Design review of the part built by this model. Coordinates are the model's own, in mm. A direction names the side the tool comes from. Give positions to 0.01 mm unless a question says otherwise; leave off trailing zeros. Write each loop counter-clockwise with the first axis right and the second up, starting at its lowest first coordinate (ties: lowest second). Pieces come first, ordered by that corner, then holes. Notation, with made-up numbers: M 83,-17 L 96,-17 A31 cw 96,20 Z; hole C 84,73 d4. An arc over 180 degrees is marked long. Answer in a Markdown table with one row per item.
```python
from build123d import *

# Parameters (mm, degrees)
EXTRUDE_1_DEPTH     = 10
FILLET_1_R          = 10
CUT_EXTRUDE_1_DEPTH = 211.475651798
CUT_EXTRUDE_2_DEPTH = 7
SKETCH_4_W          = 20.2
SKETCH_4_H          = 40
CUT_EXTRUDE_3_DEPTH = 7
CUT_EXTRUDE_4_DEPTH = 7


with BuildPart() as part:
    # Эскиз1 → Бобышка-Вытянуть1 (new body)
    with BuildSketch(Plane.XY):
        Polygon((0, 0), (60, 0), (60, -60), (90, -70.919107028), (90, -129.080892972), (60, -140), (60, -180), (0, -180), (0, -140), (-30, -129.080892972), (-30, -70.919107028), (0, -60), align=None)
    extrude(amount=EXTRUDE_1_DEPTH)

    # Скругление1
    fillet_1_edges = [part.edges().sort_by_distance(p)[0] for p in [
        (60, -60, 5),
        (90, -70.919107028, 5),
        (90, -129.080892972, 5),
        (60, -140, 5),
        (60, -180, 5),
        (0, -180, 5),
        (0, -140, 5),
        (-30, -129.080892972, 5),
        (-30, -70.919107028, 5),
        (0, -60, 5),
    ]]
    fillet(fillet_1_edges, radius=FILLET_1_R)

    # Эскиз2 → Вырез-Вытянуть1 (cut, through all)
    with BuildSketch(Plane(origin=(0, 10, 10), x_dir=(-1, 0, 0), z_dir=(0, 0, 1))):
        with BuildLine():
            Line((20, 102.25), (-80, 102.25))
            ThreePointArc((-80, 102.25), (-83.25, 99), (-80, 95.75))
            Line((-80, 95.75), (20, 95.75))
            ThreePointArc((20, 95.75), (23.25, 99), (20, 102.25))
        make_face()
        with BuildLine():
            Line((20, 91.25), (-80, 91.25))
            ThreePointArc((-80, 91.25), (-83.25, 88), (-80, 84.75))
            Line((-80, 84.75), (20, 84.75))
            ThreePointArc((20, 84.75), (23.25, 88), (20, 91.25))
        make_face()
        with BuildLine():
            Line((20, 113.25), (-80, 113.25))
            ThreePointArc((-80, 113.25), (-83.25, 110), (-80, 106.75))
            Line((-80, 106.75), (20, 106.75))
            ThreePointArc((20, 106.75), (23.25, 110), (20, 113.25))
        make_face()
        with BuildLine():
            Line((20, 124.25), (-80, 124.25))
            ThreePointArc((-80, 124.25), (-83.25, 121), (-80, 117.75))
            Line((-80, 117.75), (20, 117.75))
            ThreePointArc((20, 117.75), (23.25, 121), (20, 124.25))
        make_face()
        with BuildLine():
            Line((20, 135.25), (-80, 135.25))
            ThreePointArc((-80, 135.25), (-83.25, 132), (-80, 128.75))
            Line((-80, 128.75), (20, 128.75))
            ThreePointArc((20, 128.75), (23.25, 132), (20, 135.25))
        make_face()
    extrude(amount=-CUT_EXTRUDE_1_DEPTH, mode=Mode.SUBTRACT)

    # Эскиз3 → Вырез-Вытянуть2 (cut)
    with BuildSketch(Plane(origin=(0, 0, 0), x_dir=(-1, 0, 0), z_dir=(0, 0, -1))):
        Polygon((-57, -137.899377385), (-3, -137.899377385), (27, -126.980270357), (27, -73.019729643), (-3, -62.100622615), (-57, -62.100622615), (-87, -73.019729643), (-87, -126.980270357), align=None)
    extrude(amount=-CUT_EXTRUDE_2_DEPTH, mode=Mode.SUBTRACT)

    # Эскиз4 → Вырез-Вытянуть3 (cut)
    with BuildSketch(Plane(origin=(0, 0, 0), x_dir=(-1, 0, 0), z_dir=(0, 0, -1))):
        with Locations((-30, -44.75)):
            Rectangle(SKETCH_4_W, SKETCH_4_H)
    extrude(amount=-CUT_EXTRUDE_3_DEPTH, mode=Mode.SUBTRACT)

    # Эскиз6 → Вырез-Вытянуть4 (cut)
    with BuildSketch(Plane(origin=(0, 0, 0), x_dir=(-1, 0, 0), z_dir=(0, 0, -1))):
        with BuildLine():
            Line((-57, -135), (-57, -170))
            ThreePointArc((-57, -170), (-53.85, -173.15), (-50.7, -170))
            Line((-50.7, -170), (-50.7, -135))
            ThreePointArc((-50.7, -135), (-53.85, -131.85), (-57, -135))
        make_face()
        with BuildLine():
            Line((-47.46, -135), (-47.46, -170))
            ThreePointArc((-47.46, -170), (-44.31, -173.15), (-41.16, -170))
            Line((-41.16, -170), (-41.16, -135))
            ThreePointArc((-41.16, -135), (-44.31, -131.85), (-47.46, -135))
        make_face()
        with BuildLine():
            Line((-37.92, -135), (-37.92, -170))
            ThreePointArc((-37.92, -170), (-34.77, -173.15), (-31.62, -170))
            Line((-31.62, -170), (-31.62, -135))
            ThreePointArc((-31.62, -135), (-34.77, -131.85), (-37.92, -135))
        make_face()
        with BuildLine():
            Line((-28.38, -135), (-28.38, -170))
            ThreePointArc((-28.38, -170), (-25.23, -173.15), (-22.08, -170))
            Line((-22.08, -170), (-22.08, -135))
            ThreePointArc((-22.08, -135), (-25.23, -131.85), (-28.38, -135))
        make_face()
        with BuildLine():
            Line((-18.84, -135), (-18.84, -170))
            ThreePointArc((-18.84, -170), (-15.69, -173.15), (-12.54, -170))
            Line((-12.54, -170), (-12.54, -135))
            ThreePointArc((-12.54, -135), (-15.69, -131.85), (-18.84, -135))
        make_face()
        with BuildLine():
            Line((-9.3, -135), (-9.3, -170))
            ThreePointArc((-9.3, -170), (-6.15, -173.15), (-3, -170))
            Line((-3, -170), (-3, -135))
            ThreePointArc((-3, -135), (-6.15, -131.85), (-9.3, -135))
        make_face()
    extrude(amount=-CUT_EXTRUDE_4_DEPTH, mode=Mode.SUBTRACT)


solid = part.part
```
1) To check wall thickness, follow probe 1 along Y at (x, z) = (23, 7.5); probe 2 along X at (y, z) = (-46, 3.5); probe 3 along Y at (x, z) = (69, 8). State the ranges of each line that lie inside material, in increasing order. Write a range as [from, to].
Geometry says:
| item | result |
|---|---|
| probe 1 | [-180, -125.25], [-118.75, -114.25], [-107.75, -103.25], [-96.75, -92.25], [-85.75, -81.25], [-74.75, 0] |
| probe 2 | [0, 19.9], [40.1, 60] |
| probe 3 | [-136.72, -125.25], [-118.75, -114.25], [-107.75, -103.25], [-96.75, -92.25], [-85.75, -81.25], [-74.75, -63.28] |
2) Insertion check: P1, Ø5.5, axis at y = -150.5, z = 3.5, coming from the +X side; P2, Ø5, axis at y = -54, z = 3.5, coming from the -X side; P3, Ø1.5, axis at x = 55, z = 5, coming from the +Y side; P4, Ø10, axis at x = 40.5, y = -73, coming from the -Z side. Each pin has a flat end and moves straight along its axis. Give the tip position at first contact, or say it passes through.
Geometry says:
| item | result |
|---|---|
| P1 | x = 60 |
| P2 | x = -0.63 |
| P3 | y = 0 |
| P4 | z = 7 |
3) Add section A-A (x = 34.77). Write out the cut boundary in (y, z), and give its area (3 significant figures).
Geometry says:
| item | result |
|---|---|
| outline | M -180,0 L -173.15,0 L -173.15,7 L -125.25,7 L -125.25,10 L -180,10 Z; M -118.75,7 L -114.25,7 L -114.25,10 L -118.75,10 Z; M -107.75,7 L -103.25,7 L -103.25,10 L -107.75,10 Z; M -96.75,7 L -92.25,7 L -92.25,10 L -96.75,10 Z; M -85.75,7 L -81.25,7 L -81.25,10 L -85.75,10 Z; M -74.75,7 L -24.75,7 L -24.75,0 L 0,0 L 0,10 L -74.75,10 Z |
| area | 664 mm^2 |
4) The part is to be moulded in two halves that separate along Y. For faces 4 (the face through (30, 0, 5)), 5 (the face through (34.84, -173.15, 3.45)), 6 (the face through (30, -24.75, 3)), 7 (the face through (60, -158, 5)), say which applies: released by +Y, released by -Y, zero draft, split by the parting line, or undercut.
Geometry says:
| item | result |
|---|---|
| face 4 | released by +Y |
| face 5 | undercut |
| face 6 | undercut |
| face 7 | zero draft |
5) Add section D-D (y = -17). Write out the cut boundary in (x, z), and give its area (3 significant figures).
Geometry says:
| item | result |
|---|---|
| outline | M 0,0 L 60,0 L 60,10 L 0,10 Z |
| area | 600 mm^2 |
6) Add section B-B (y = -100). Write out the cut boundary in (x, z).
Geometry says:
| item | result |
|---|---|
| outline | M -30,0 L -27,0 L -27,7 L -23.25,7 L -23.25,10 L -30,10 Z; M 83.25,7 L 87,7 L 87,0 L 90,0 L 90,10 L 83.25,10 Z |
7) Add section C-C (x = 70.5). Write out the cut boundary in (y, z).
Geometry says:
| item | result |
|---|---|
| outline | M -136.18,0 L -132.99,0 L -132.99,7 L -125.25,7 L -125.25,10 L -136.18,10 Z; M -118.75,7 L -114.25,7 L -114.25,10 L -118.75,10 Z; M -107.75,7 L -103.25,7 L -103.25,10 L -107.75,10 Z; M -96.75,7 L -92.25,7 L -92.25,10 L -96.75,10 Z; M -85.75,7 L -81.25,7 L -81.25,10 L -85.75,10 Z; M -74.75,7 L -67.01,7 L -67.01,0 L -63.82,0 L -63.82,10 L -74.75,10 Z |
8) For faces 1 (the face through (18.84, -154, 3)), 2 (the face through (83.25, -111.07, 8.52)), 3 (the face through (-2, -141, 5)), list the 3-axis set-ups (+Z, -Z, +X, -X, +Y, -Y) from which the entire face can be reached by the end or side of a thin tool; tool diameter is ignored.
Geometry says:
| item | result |
|---|---|
| face 1 | -Z |
| face 2 | +Z, -Z |
| face 3 | +Z, -Z, -X, -Y |
